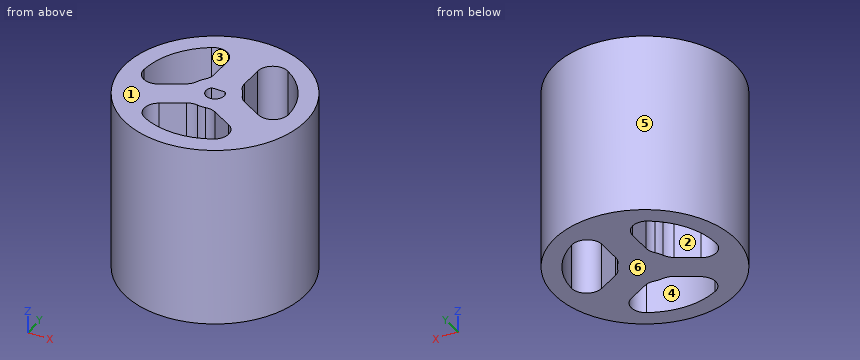
```python
from build123d import *

# Parameters (mm, degrees)
SZKIC1_R                        = 30
DODANIE_WYCI_GNI_CIE1_DEPTH     = 60
WYTNIJ_WYCI_GNI_CIE1_DEPTH      = 74.484692283
WYTNIJ_WYCI_GNI_CIE1_DEPTH_BACK = 13
WYTNIJ_WYCI_GNI_CIE4_DEPTH      = 74.484692283
ZAOKR_GLENIE2_R                 = 5


with BuildPart() as part:
    # Szkic1 → Dodanie-wyciągnięcie1 (new body)
    with BuildSketch(Plane.XY):
        Circle(SZKIC1_R)
    extrude(amount=DODANIE_WYCI_GNI_CIE1_DEPTH)

    # Szkic3 → Wytnij-wyciągnięcie1 (cut, two sides: drawn at the far end of the back side and taken through both)
    with BuildSketch(Plane.XY.offset(60).offset(-WYTNIJ_WYCI_GNI_CIE1_DEPTH_BACK)):
        with BuildLine():
            Line((2.224367528, 2.013004993), (-2.224367528, 2.013004993))
            ThreePointArc((-2.224367528, 2.013004993), (0, -3), (2.224367528, 2.013004993))
        make_face()
    extrude(amount=WYTNIJ_WYCI_GNI_CIE1_DEPTH + WYTNIJ_WYCI_GNI_CIE1_DEPTH_BACK, mode=Mode.SUBTRACT)

    # Szkic4 → Wytnij-wyciągnięcie4 (cut, through all)
    with BuildSketch(Plane.XY.offset(60)):
        with BuildLine():
            ThreePointArc((-7.908326913, 1.20762802), (-6.92820323, 4), (-5, 6.244997998))
            Line((-5, 6.244997998), (-5, 23.473389189))
            ThreePointArc((-5, 23.473389189), (-20.784609691, 12), (-22.82855135, -7.406567575))
            Line((-22.82855135, -7.406567575), (-7.908326913, 1.20762802))
        make_face()
        with BuildLine():
            Line((5, 23.473389189), (5, 6.244997998))
            ThreePointArc((5, 6.244997998), (6.92820323, 4), (7.908326913, 1.20762802))
            Line((7.908326913, 1.20762802), (22.82855135, -7.406567575))
            ThreePointArc((22.82855135, -7.406567575), (23.705328857, -3.749317778), (24, 0))
            ThreePointArc((24, 0), (18.654758106, 15.099668871), (5, 23.473389189))
        make_face()
        with BuildLine():
            ThreePointArc((2.908326913, -7.452626018), (0, -8), (-2.908326913, -7.452626018))
            Line((-2.908326913, -7.452626018), (-17.82855135, -16.066821613))
            ThreePointArc((-17.82855135, -16.066821613), (0, -24), (17.82855135, -16.066821613))
            Line((17.82855135, -16.066821613), (2.908326913, -7.452626018))
        make_face()
    extrude(amount=-WYTNIJ_WYCI_GNI_CIE4_DEPTH, mode=Mode.SUBTRACT)

    # Zaokrąglenie2
    zaokr_glenie2_edges = [part.edges().sort_by_distance(p)[0] for p in [
        (-17.82855135, -16.066821613, 30),
        (-2.908326913, -7.452626018, 30),
        (2.908326913, -7.452626018, 30),
        (17.82855135, -16.066821613, 30),
        (22.82855135, -7.406567575, 30),
        (7.908326913, 1.20762802, 30),
        (5, 6.244997998, 30),
        (5, 23.473389189, 30),
        (-5, 23.473389189, 30),
        (-5, 6.244997998, 30),
        (-7.908326913, 1.20762802, 30),
        (-22.82855135, -7.406567575, 30),
    ]]
    fillet(zaokr_glenie2_edges, radius=ZAOKR_GLENIE2_R)


solid = part.part
```
Here's how the part is built. I have some questions about the finished solid (model axes, mm). Face numbers are marked on the shaded views. A direction names the side the tool comes from. Coordinates: 2 decimals unless noted, no trailing zeros. Write each loop counter-clockwise with the first axis right and the second up, starting at its lowest first coordinate (ties: lowest second). Pieces come first, ordered by that corner, then holes. Notation, with made-up numbers: M 19.25,8 L 65.25,8 A16 ccw 65.25,20 Z; hole C 60.25,-30.75 d10. An arc over 180 degrees is marked long. Answer as CSV lines item,"result". Start each with the question number.
Q1. I need wall thicknesses on probe 1 along Y at (x, z) = (0, 54.5); probe 2 along Y at (x, z) = (-11.5, 11); probe 3 along X at (y, z) = (-4, 57). Which ranges of each line are inside material? Lowest first, please. Write a range as [from, to].
Q2. Suppose I cut it at A-A, the plane x = 0. List the corners of the cut face in (y, z) for me.
Q3. Will these pins go through, and if not, where does the flat tip stop? pin 1 Ø12 at (x, z) = (13.5, 52.5) entering from +Y; pin 2 Ø3 at (y, z) = (20, 14.5) entering from +X; pin 3 Ø8.5 at (y, z) = (13.5, 21) entering from -X.
Q4. If we mould it in two halves opening along Y, with no side actions, what happens to the marked faces 3, 4, 5 and 6? For each: pulls with the +Y half, pulls with the -Y half, needs draft (parallel to the pull), parting line crosses it, or undercut.
Q5. Suppose I cut it at D-D, the plane z = 49. State how many separate pieces and enclosed holes the cut face has, then the cut area to 3 significant figures.
Q6. Suppose I cut it at C-C, the plane y = 14. List the corners of the cut face in (x, z) for me.
Q7. Suppose I cut it at B-B, the plane y = -10. List the corners of the cut face in (x, z) for me, then the cut area to 3 significant figures.
Q8. For the marked faces 1 and 2, which set-ups out of +Z, -Z, +X, -X, +Y, -Y let a thin tool reach every point of the face, with its end or its side?
Entries:
1,probe 1,"y = [-30, -24], [-8, -3], [2.01, 30]"
1,probe 2,"y = [-27.71, -21.06], [-12.41, -0.87], [20.93, 27.71]"
1,probe 3,"x = [-29.73, -20.99], [-16.99, 16.99], [20.99, 29.73]"
2,outline,"M -30,0 L -24,0 L -24,60 L -30,60 Z; M -8,0 L 30,0 L 30,60 L 2.01,60 L 2.01,47 L -3,47 L -3,60 L -8,60 Z"
3,pin 1,"stops at y = 29.05"
3,pin 2,"stops at x = 23.62"
3,pin 3,"stops at x = -28.54"
4,face 3,"undercut"
4,face 4,"undercut"
4,face 5,"parting line crosses it"
4,face 6,"needs draft"
5,separate pieces,"1"
5,enclosed holes,"4"
5,area,"1,770 mm²"
6,outline,"M -26.53,0 L -19.49,0 L -19.49,60 L -26.53,60 Z; M -5,0 L 5,0 L 5,60 L -5,60 Z; M 19.49,0 L 26.53,0 L 26.53,60 L 19.49,60 Z"
7,outline,"M -28.28,0 L -7.32,0 L -7.32,60 L -28.28,60 Z; M 7.32,0 L 28.28,0 L 28.28,60 L 7.32,60 Z"
7,area,"2,520 mm²"
8,face 1,"+Z, +X, -X, +Y, -Y"
8,face 2,"+Z, -Z"
